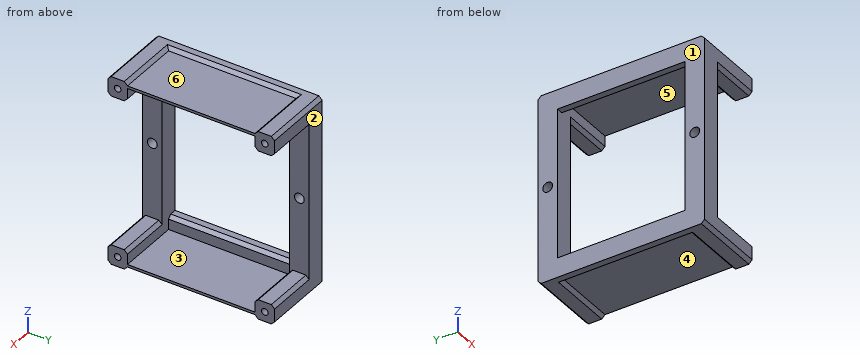
Autodesk Inventor part; units mm, degrees
ref_plane "YZ Plane" through (0, 0, 0) normal (1, 0, 0) x (0, 1, 0)
ref_plane "XZ Plane" through (0, 0, 0) normal (0, 1, 0) x (-1, 0, 0)
ref_plane "XY Plane" through (0, 0, 0) normal (0, 0, 1) x (1, 0, 0)
sketch "Sketch1" plane through (0, 0, 0) normal (0, 1, 0) x (-1, 0, 0)
  line L0 (0, 0) -> (22, 0)
  line L1 (22, 0) -> (22, -58)
  line L2 (22, -58) -> (0, -58)
  line L3 (0, -58) -> (0, -52)
  line L4 (0, -52) -> (16, -52)
  line L5 (16, -52) -> (16, -6)
  line L6 (16, -6) -> (0, -6)
  line L7 (0, -6) -> (0, 0)
  dimension "d0" = 6
  dimension "d1" = 6
  dimension "d2" = 58
  dimension "d3" = 22
extrude "Extrusion1" add sketch "Sketch1" along normal blind 6
sketch "Sketch2" plane through (0, 0, 0) normal (1, 0, 0) x (0, 0, -1)
  line L0 (6, 6) -> (52, 6)
  line L1 (0, 0) -> (6, 6) construction
  line L2 (58, 0) -> (58, 6)
  line L3 (52, 6) -> (58, 0) construction
  circle A0 centre (3, 3) radius 1
  circle A1 centre (55, 3) radius 1
  dimension "d6" = 2
extrude "Extrusion2" cut sketch "Sketch2" against normal blind 12
sketch "Sketch3" plane through (-16, 0, -6) normal (1, 0, 0) x (0, 0, -1)
  line L0 (0, 6) -> (46, 6)
  line L1 (23, 6) -> (23, 0) construction
  circle A0 centre (23, 3) radius 1.5
  line L2 (0, 0) -> (46, 0)
  point P0 (-6, 0)
  dimension "d9" = 3
extrude "Extrusion3" cut sketch "Sketch3" against normal through all
pattern_linear "Rectangular Pattern2" count 2 spacing 45 along (0, 1, 0) of "Extrusion1", "Extrusion3", "Extrusion2"
sketch "Sketch5" plane through (-22, 0, -58) normal (-1, 0, 0) x (0, 0, 1)
  line L0 (58, 0) -> (52, 0)
  line L1 (52, 51) -> (6, 51)
  line L2 (58, 0) -> (52, 0)
  line L3 (52, 0) -> (52, 51)
  line L4 (52, 51) -> (58, 51)
  line L5 (58, 51) -> (58, 0)
  line L6 (6, 0) -> (0, 0)
  line L7 (6, 45) -> (6, 51)
  line L8 (0, 0) -> (6, 0)
  line L9 (6, 0) -> (6, 51)
  line L10 (6, 51) -> (0, 51)
  line L11 (0, 51) -> (0, 0)
extrude "Extrusion4" add sketch "Sketch5" against normal blind 3
chamfer "Chamfer3" distance 1 angle 45 20 edges at (-11, 51, 0) (-9.5, 45, 0) (-8, 51, -6) (-8, 45, -52) (-8, 51, -52) (-11, 51, -58) (-9.5, 6, -58) (-8, 6, -52) (-8, 0, -52) (-8, 6, -6) (-9.5, 6, 0) (-11, 0, 0) (-8, 45, -6) (-8, 0, -6) (-11, 0, -58) (-9.5, 45, -58) (-19, 25.5, -6) (-19, 25.5, 0) (-19, 25.5, -52) (-19, 25.5, -58)
sketch "Sketch6" plane through (0, 45, -1) normal (1, 0, 0) x (0, 0, -1)
  point P0 (-1, -45)
sketch "Sketch7" plane through (0, 45, -53) normal (1, 0, 0) x (0, 0, -1)
  line L0 (-52, 0) -> (-48, 0)
  line L1 (-52, -39) -> (-48, -39)
  line L2 (-52, 0) -> (-51.2, 0)
  line L3 (-51.2, 0) -> (-51.2, -39)
  line L4 (-51.2, -39) -> (-52, -39)
  line L5 (-52, -39) -> (-52, 0)
  line L6 (0, 0) -> (4, 0)
  line L7 (4, 0) -> (3.2, 0)
  line L8 (3.2, 0) -> (3.2, -39)
  line L9 (3.2, -39) -> (4, -39)
  line L10 (4, -39) -> (4, 0)
  line L11 (0, -39) -> (4, -39)
  point P0 (-53, -45)
  point P1 (3.2, 0)
  dimension "d29" = 0.8
  dimension "d30" = 0.8
extrude "Extrusion5" add sketch "Sketch7" against normal up to surface (19 mm away)
equation "\"d30\" = d29"
properties part number "batt-standoff"
Geometry: final body of the model. Coordinates: model frame, mm. Face numbers are marked on the shaded views. A direction names the side the tool comes from. Round coordinates to 2 decimals unless told otherwise and drop trailing zeros. Write each loop counter-clockwise with the first axis right and the second up, starting at its lowest first coordinate (ties: lowest second). Pieces come first, ordered by that corner, then holes. Notation, with made-up numbers: M -34,72 L -24,72 A22 ccw -24,100 Z; hole C 74.25,-8.5 d7. An arc over 180 degrees is marked long. Write item = value, one per line.
Item 1: Section query B-B on z = -50.5. Return loops of the section in (x, y), then the cut area to 3 significant figures.
Findings:
outline = M -22,0 L -16,0 L -16,6 L -22,6 Z; M -22,45 L -16,45 L -16,51 L -22,51 Z
area = 72.0 mm^2
Item 2: Pin query (flat end, axial travel): P1, Ø5, axis at x = -12.5, y = 34.5, coming from the -Z side; P2, Ø11, axis at x = -7, z = -24.5, coming from the -Y side; P3, Ø4, axis at y = 3, z = -29, coming from the +X side; P4, Ø2, axis at x = -6, y = 21, coming from the +Z side. Return the tip coordinate at first contact, or that it passes through.
Findings:
P1 = -57
P2 = through
P3 = -16
P4 = -1
Item 3: Material intervals for line 1 along Y through (x, z) = (-19.5, -51); line 2 along Y through (x, z) = (-5.25, -3); line 3 along Y through (x, z) = (-18.5, -29), sorted ascending. Write a range as [from, to].
Findings:
line_1 = [0, 6], [45, 51]
line_2 = [0, 2], [4, 6], [45, 47], [49, 51]
line_3 = [0, 1.5], [4.5, 6], [45, 46.5], [49.5, 51]
Item 4: Section query C-C on z = -29. Return loops of the section in (x, y), then the cut area to 3 significant figures.
Findings:
outline = M -22,0 L -16,0 L -16,1.5 L -22,1.5 Z; M -22,4.5 L -16,4.5 L -16,6 L -22,6 Z; M -22,45 L -16,45 L -16,46.5 L -22,46.5 Z; M -22,49.5 L -16,49.5 L -16,51 L -22,51 Z
area = 36.0 mm^2
Item 5: Section query A-A on y = 31. Return loops of the section in (x, z).
Findings:
outline = M -22,-58 L -20,-58 L -19,-57 L 0,-57 L 0,-56.2 L -19,-56.2 L -19,-53 L -20,-52 L -22,-52 Z; M -22,-6 L -20,-6 L -19,-5 L -19,-1.8 L 0,-1.8 L 0,-1 L -19,-1 L -20,0 L -22,0 Z
Item 6: Access query for the marked faces 4, 5 and 6. Directions: +Z, -Z, +X, -X, +Y, -Y. A direction counts if a zero-diameter tool reaches every point of the face in a straight line with its end or side. Return the directions, or none.
Findings:
face_4 = -Z, +X
face_5 = +X
face_6 = +Z, +X
Item 7: Section query D-D on x = -2.75. State how many separate pieces and enclosed holes the cut face has, then the cut area to 3 significant figures.
Findings:
separate_pieces = 2
enclosed_holes = 4
area = 186 mm^2
Item 8: Pull-direction query (Y, two-part tool) for the marked faces 1, 2 and 3; classes: pulls with the +Y half, pulls with the -Y half, needs draft (parallel to the pull), parting line crosses it, or undercut.
Findings:
face_1 = needs draft
face_2 = pulls with the +Y half
face_3 = undercut
